Source: CAD feature listing. Evaluate the final solid. Frame: model axes, mm. A direction names the side the tool comes from. Round coordinates to 2 decimals unless told otherwise and drop trailing zeros. Order: outer loops, then holes, each group sorted by start corner. A loop starts at its lowest first (then second) coordinate and runs counter-clockwise, first axis right, second up. Notation, with made-up numbers: (67.5, 14) -> (113.5, 14) arc R36 cw to (113.5, 52) -> close; hole circle Ø6 at (8, -24.75). An arc over 180 degrees is marked (long way). Use a Markdown table: item, result. Add a question column.
Autodesk Inventor part; units mm, degrees
ref_plane "YZ Plane" through (0, 0, 0) normal (1, 0, 0) x (0, 1, 0)
ref_plane "XZ Plane" through (0, 0, 0) normal (0, 1, 0) x (-1, 0, 0)
ref_plane "XY Plane" through (0, 0, 0) normal (0, 0, 1) x (1, 0, 0)
sketch "Sketch1" plane through (0, 0, 0) normal (0, 0, 1) x (1, 0, 0)
  circle A0 centre (0, 0) radius 4
  circle A1 centre (0, 0) radius 8
  circle A2 centre (0, 0) radius 12
  dimension "d0" = 8
  dimension "d1" = 16
  dimension "d2" = 24
extrude "Extrusion1" add sketch "Sketch1" along normal mid plane 4 contours A1
sketch "Sketch2" plane through (0, 0, 2) normal (0, 0, 1) x (1, 0, 0)
  circle A0 centre (0, 0) radius 12
  circle A1 centre (0, 0) radius 8
extrude "Extrusion2" add sketch "Sketch2" along normal blind 2 contours A0 | A1
mirror "Mirror1" about plane through (0, 0, 0) normal (0, 0, 1) of "Extrusion2"
extrude "Extrusion3" cut sketch "Sketch1" along normal through all both and the other way through all contours A0
sketch "Sketch3" plane through (0, 0, -4) normal (0, 0, -1) x (-1, 0, 0)
  circle A0 centre (0, 0) radius 7
  line L0 (0, -7) -> (0, 7)
  circle A1 centre (0, -7) radius 1
  circle A2 centre (0, 7) radius 1
  dimension "d9" = 14
  dimension "d10" = 2
  dimension "d11" = 2
extrude "Extrusion4" cut sketch "Sketch3" against normal through all contours A2 L0 A0 | A0 A2 | A1 A0 | A0 L0 A1 | L0 A2 A0 | A0 A1 L0
pattern_circular "Circular Pattern1" count 4 over 360 about axis through (0, 0, -10) along (0, 0, 1) of "Extrusion4"
properties part number "Servo Pulley"
1) Draft query along Z for faces 1 (the cylindrical face through (-1.73, -7.81, 0.03)), 2 (the flat face through (3, 3, -4)), 3 (the flat face through (-3, 3, 4)), 4 (the cylindrical face through (-11.99, -0.53, 2.99)). Return one class per face: pulls with the +Z half, pulls with the -Z half, needs draft (parallel to the pull), parting line crosses it, or undercut.
2) Section B-B on z = -3. Output: boundary loops of the cut face in (x, y), then the cut area to 3 significant figures.
3) Reachability of faces 5 (the flat face through (2, -8, 2)), 6 (the cylindrical face through (-7.676, 0.737, -0.056)) from +Z, -Z, +X, -X, +Y, -Y: full face, straight path, thin tool, end or side. Return the list, or none.
4) Section C-C on y = -3.5. Output: boundary loops of the cut face in (x, z).
5) First-contact query: pin 1 Ø1.2 at (x, y) = (-7, 0) entering from +Z; pin 2 Ø3 at (x, y) = (7, 0) entering from +Z; pin 3 Ø1 at (y, z) = (-5, 3) entering from -X; pin 4 Ø4 at (y, z) = (9, 3) entering from +X. Flat tips, straight axial feed; report the tip coordinate or a pass-through.
6) Section A-A on x = -7. Output: boundary loops of the cut face in (y, z), then the cut area to 3 significant figures.
7) Line query: probe 1 along Z at (x, y) = (11, -3.5); probe 2 along X at (y, z) = (7.25, -3.5); probe 3 along Y at (x, z) = (-6.75, -2.5). Output: solid intervals per line, ascending. Write a range as from..to.
8) Section D-D on x = -0.25. Output: boundary loops of the cut face in (y, z).
Conclusion:
| question | item | result |
|---|---|---|
| 1 | face 1 | undercut |
| 1 | face 2 | pulls with the -Z half |
| 1 | face 3 | pulls with the +Z half |
| 1 | face 4 | needs draft |
| 2 | outline | circle Ø24 at (0, 0); hole circle Ø2 at (-7, 0); hole circle Ø8 at (0, 0); hole circle Ø2 at (0, -7); hole circle Ø2 at (0, 7); hole circle Ø2 at (7, 0) |
| 2 | area | 390 mm^2 |
| 3 | face 5 | none |
| 3 | face 6 | +Z, -Z |
| 4 | outline | (-11.48, -4) -> (-1.94, -4) -> (-1.94, 4) -> (-11.48, 4) -> (-11.48, 2) -> (-7.19, 2) -> (-7.19, -2) -> (-11.48, -2) -> close; (1.94, -4) -> (11.48, -4) -> (11.48, -2) -> (7.19, -2) -> (7.19, 2) -> (11.48, 2) -> (11.48, 4) -> (1.94, 4) -> close |
| 5 | pin 1 | passes through |
| 5 | pin 2 | stops at z = 4 |
| 5 | pin 3 | stops at x = -11.12 |
| 5 | pin 4 | stops at x = 9.75 |
| 6 | outline | (-9.75, -4) -> (-1, -4) -> (-1, 4) -> (-9.75, 4) -> (-9.75, 2) -> (-3.87, 2) -> (-3.87, -2) -> (-9.75, -2) -> close; (1, -4) -> (9.75, -4) -> (9.75, -2) -> (3.87, -2) -> (3.87, 2) -> (9.75, 2) -> (9.75, 4) -> (1, 4) -> close |
| 6 | area | 93.0 mm^2 |
| 7 | probe 1 | z = -4..-2, 2..4 |
| 7 | probe 2 | x = -9.56..-0.97, 0.97..9.56 |
| 7 | probe 3 | y = -9.92..-0.97, 0.97..9.92 |
| 8 | outline | (-12, -4) -> (-7.97, -4) -> (-7.97, 4) -> (-12, 4) -> (-12, 2) -> (-8, 2) -> (-8, -2) -> (-12, -2) -> close; (-6.03, -4) -> (-3.99, -4) -> (-3.99, 4) -> (-6.03, 4) -> close; (3.99, -4) -> (6.03, -4) -> (6.03, 4) -> (3.99, 4) -> close; (7.97, -4) -> (12, -4) -> (12, -2) -> (8, -2) -> (8, 2) -> (12, 2) -> (12, 4) -> (7.97, 4) -> close |
